Here's how the part is built. I have some questions about the finished solid (model axes, mm). A direction names the side the tool comes from. Coordinates: 2 decimals unless noted, no trailing zeros. Order: outer loops, then holes, each group sorted by start corner. A loop starts at its lowest first (then second) coordinate and runs counter-clockwise, first axis right, second up.
```python
from build123d import *

# Parameters (mm, degrees)
BOSS_EXTRUDE2_DEPTH = 10
BOSS_EXTRUDE4_DEPTH = 60
SKETCH4_R           = 5.950427228
SKETCH4_R_2         = 3.640178542
BOSS_EXTRUDE5_DEPTH = 5
SKETCH9_R           = 17.396356036
SKETCH9_R_2         = 12.893034815
BOSS_EXTRUDE7_DEPTH = 50
SKETCH11_R          = 12.893034815
CUT_EXTRUDE2_DEPTH  = 96.902358539
SKETCH12_R          = 3.108842341
CUT_EXTRUDE5_DEPTH  = 63
SKETCH16_R          = 3.004688719
CUT_EXTRUDE6_DEPTH  = 66


with BuildPart() as part:
    # Sketch1 → Boss-Extrude2 (new body)
    with BuildSketch(Plane(origin=(0, 0, 0), x_dir=(1, 0, 0), z_dir=(0, 1, 0))):
        with BuildLine():
            Line((-38.603351955, 28.351955307), (41.396648045, 28.351955307))
            ThreePointArc((41.396648045, 28.351955307), (48.467715857, 25.423023119), (51.396648045, 18.351955307))
            Line((51.396648045, 18.351955307), (51.396648045, -11.648044693))
            ThreePointArc((51.396648045, -11.648044693), (48.467715857, -18.719112505), (41.396648045, -21.648044693))
            Line((41.396648045, -21.648044693), (-38.603351955, -21.648044693))
            ThreePointArc((-38.603351955, -21.648044693), (-45.674419767, -18.719112505), (-48.603351955, -11.648044693))
            Line((-48.603351955, -11.648044693), (-48.603351955, 18.351955307))
            ThreePointArc((-48.603351955, 18.351955307), (-45.674419767, 25.423023119), (-38.603351955, 28.351955307))
        make_face()
    extrude(amount=BOSS_EXTRUDE2_DEPTH)

    # Sketch3 → Boss-Extrude4 (add)
    with BuildSketch(Plane(origin=(0, 10, 0), x_dir=(1, 0, 0), z_dir=(0, 1, 0))):
        with BuildLine():
            Line((-23.603351955, 10.851955307), (26.396648045, 10.851955307))
            ThreePointArc((26.396648045, 10.851955307), (29.932181951, 9.387489213), (31.396648045, 5.851955307))
            Line((31.396648045, 5.851955307), (31.396648045, 0.851955307))
            ThreePointArc((31.396648045, 0.851955307), (29.932181951, -2.683578599), (26.396648045, -4.148044693))
            Line((26.396648045, -4.148044693), (-23.603351955, -4.148044693))
            ThreePointArc((-23.603351955, -4.148044693), (-27.138885861, -2.683578599), (-28.603351955, 0.851955307))
            Line((-28.603351955, 0.851955307), (-28.603351955, 5.851955307))
            ThreePointArc((-28.603351955, 5.851955307), (-27.138885861, 9.387489213), (-23.603351955, 10.851955307))
        make_face()
    extrude(amount=BOSS_EXTRUDE4_DEPTH)

    # Sketch4 → Boss-Extrude5 (add)
    # profile 1 of 2: a face of its own
    with BuildSketch(Plane(origin=(0, 10, 0), x_dir=(1, 0, 0), z_dir=(0, 1, 0))):
        with Locations((34.396648045, -4.648044693)):
            Circle(SKETCH4_R)
        with Locations(Location((34.396648045, -4.648044693, 0), (0, 0, 270))):
            Circle(SKETCH4_R_2, mode=Mode.SUBTRACT)
    # profile 2 of 2: a face of its own
    with BuildSketch(Plane(origin=(0, 10, 0), x_dir=(1, 0, 0), z_dir=(0, 1, 0))):
        with Locations((-31.603351955, -4.648044693)):
            Circle(SKETCH4_R)
        with Locations(Location((-31.603351955, -4.648044693, 0), (0, 0, 90))):
            Circle(SKETCH4_R_2, mode=Mode.SUBTRACT)
    extrude(amount=BOSS_EXTRUDE5_DEPTH)

    # Sketch9 → Boss-Extrude7 (add)
    with BuildSketch(Plane.XY.offset(14.148044693)):
        with Locations((1.396648045, 53)):
            Circle(SKETCH9_R)
        with Locations((1.396648045, 53)):
            Circle(SKETCH9_R_2, mode=Mode.SUBTRACT)
    extrude(amount=-BOSS_EXTRUDE7_DEPTH)

    # Sketch11 → Cut-Extrude2 (cut, through all)
    with BuildSketch(Plane.XY.offset(4.148044693)):
        with Locations((1.396648045, 53)):
            Circle(SKETCH11_R)
    extrude(amount=-CUT_EXTRUDE2_DEPTH, mode=Mode.SUBTRACT)

    # Sketch12 → Cut-Extrude5 (cut)
    with BuildSketch(Plane(origin=(0, 70, 0), x_dir=(1, 0, 0), z_dir=(0, 1, 0))):
        with Locations(Location((26.396648045, 2.851955307, 0), (0, 0, 270))):
            Circle(SKETCH12_R)
        with Locations(Location((-23.603351955, 2.851955307, 0), (0, 0, 90))):
            Circle(SKETCH12_R)
    extrude(amount=-CUT_EXTRUDE5_DEPTH, mode=Mode.SUBTRACT)

    # Sketch16 → Cut-Extrude6 (cut)
    with BuildSketch(Plane(origin=(0, 75, 0), x_dir=(1, 0, 0), z_dir=(0, 1, 0))):
        with Locations(Location((1.396648045, 2.996607423, 0), (0, 0, 270))):
            Circle(SKETCH16_R)
    extrude(amount=-CUT_EXTRUDE6_DEPTH, mode=Mode.SUBTRACT)


solid = part.part
```
Q1. If we section it at A-A on y = 53: Write out the boundary of the cut face in (x, z).
Q2. If we section it at D-D on z = -20: Write out the boundary of the cut face in (x, y), then the cut area to 3 significant figures.
Q3. If we section it at B-B on z = -12.5: Write out the boundary of the cut face in (x, y), then the cut area to 3 significant figures.
Q4. If we section it at C-C on x = -9.5: Write out the boundary of the cut face in (y, z), then the cut area to 3 significant figures.
Q5. I need wall thicknesses on L1, parallel to Y at x = 2, z = -18; L2, parallel to Y at x = 12, z = 8; L3, parallel to X at y = 45.5, z = -5.5. Which ranges of each line are inside material? Lowest first, please.
Q6. Will these pins go through, and if not, where does the flat tip stop? pin 1 (1.5 mm diameter, centred on y = 39, z = -3.5, fed in from -X); pin 2 (2 mm diameter, centred on x = -5.5, y = 7, fed in from -Z); pin 3 (2 mm diameter, centred on x = -32.5, z = 4.5, fed in from +Y).
Q7. We'd pull the mould along Y, two halves only. Please class faces 5 (the cylindrical face through (-27.178, 39.58, -9.348)), 6 (the flat face through (2, 0, -4)), 7 (the flat face through (2, 33, 4.148)), 8 (the flat face through (1, 9, -3)): pulls with the +Y half, pulls with the -Y half, needs draft (parallel to the pull), parting line crosses it, or undercut.
Q8. For faces 1 (the flat face through (1, 33, -10.852)), 2 (the cylindrical face through (1.5, 68, -6)), 3 (the flat face through (1, 5, -28.352)), 4 (the flat face through (-15, 70, -3)), which set-ups out of +Z, -Z, +X, -X, +Y, -Y let a thin tool reach every point of the face, with its end or its side?
Reply:
1. outline: (-28.6, -5.85) arc R5 ccw to (-23.6, -10.85) - (-16, -10.85) - (-16, -35.85) - (-11.5, -35.85) - (-11.5, 14.15) - (-16, 14.15) - (-16, 4.15) - (-23.6, 4.15) arc R5 ccw to (-28.6, -0.85) - close; (14.29, -35.85) - (18.79, -35.85) - (18.79, -10.85) - (26.4, -10.85) arc R5 ccw to (31.4, -5.85) - (31.4, -0.85) arc R5 ccw to (26.4, 4.15) - (18.79, 4.15) - (18.79, 14.15) - (14.29, 14.15) - close; hole circle Ø6.22 at (-23.6, -2.85); hole circle Ø6.22 at (26.4, -2.85)
2. outline: (-48.47, 0) - (51.26, 0) - (51.26, 10) - (-48.47, 10) - close; circle Ø34.79 at (1.4, 53); hole circle Ø25.79 at (1.4, 53)
2. area: 1,430 mm2
3. outline: (-48.6, 0) - (51.4, 0) - (51.4, 10) - (-48.6, 10) - close; circle Ø34.79 at (1.4, 53); hole circle Ø25.79 at (1.4, 53)
3. area: 1,430 mm2
4. outline: (0, -28.35) - (10, -28.35) - (10, -10.85) - (39.44, -10.85) - (39.44, -35.85) - (46.11, -35.85) - (46.11, 14.15) - (39.44, 14.15) - (39.44, 4.15) - (10, 4.15) - (10, 21.65) - (0, 21.65) - close; (59.89, -35.85) - (66.56, -35.85) - (66.56, -10.85) - (70, -10.85) - (70, 4.15) - (66.56, 4.15) - (66.56, 14.15) - (59.89, 14.15) - close
4. area: 1,660 mm2
5. L1: y = 0 to 10, 35.61 to 40.12, 65.88 to 70.39
5. L2: y = 0 to 10, 39.21 to 45.67, 60.33 to 66.79
5. L3: x = -28.6 to -25.23, -21.97 to -9.09, 11.88 to 24.77, 28.03 to 31.4
6. pin 1: stops at x = -28.6
6. pin 2: stops at z = -28.35
6. pin 3: stops at y = 10
7. face 5: needs draft
7. face 6: pulls with the -Y half
7. face 7: undercut
7. face 8: pulls with the +Y half
8. face 1: -Z
8. face 2: +Y
8. face 3: -Z, +X, -X, -Y
8. face 4: +Z, -Z, -X, +Y
